Read the model definition and answer for the solid it produces. Units are mm, in the model's axes. A direction names the side the tool comes from. Give positions to 0.01 mm unless a question says otherwise; leave off trailing zeros. Write each loop counter-clockwise with the first axis right and the second up, starting at its lowest first coordinate (ties: lowest second). Pieces come first, ordered by that corner, then holes. Notation, with made-up numbers: M 17,71.25 L 52,71.25 A16 ccw 52,84.25 Z; hole C -6,12 d6. An arc over 180 degrees is marked long. Use a Markdown table: item, result. Add a question column.
Item 1: A cutting plane is placed at C-C on y = 28. Determine the outline of the cut face in (x, z) (3 decimals), then the cut area to 3 significant figures.
Item 2: For faces 1 (the flat face through (-40.64, 0, 19)), 2 (the flat face through (48, 12.7, 19)), 3 (the flat face through (62.23, 21, 19)), 4 (the flat face through (-55, 3.175, 19)), 5 (the cylindrical face through (-62.68, 8.18, 26.34)), determine the directions among +Z, -Z, +X, -X, +Y, -Y from which every point of the face is accessible in a straight line to the end or side of a thin tool.
Item 3: Consider probe 1 along X at (y, z) = (-6, 8.5) (3 decimals); probe 2 along Y at (x, z) = (0.5, 3.5) (3 decimals); probe 3 along X at (y, z) = (8.5, 27). Determine where each line is inside the solid, lowest interval first. Write a range as [from, to].
Item 4: The mould has two halves that part along X. Classify faces 6 (the flat face through (2, -17.78, 19)), 7 (the flat face through (1, -27.305, 19)), 8 (the flat face through (-50.165, -5, 19)): pulls with the +X half, pulls with the -X half, needs draft (parallel to the pull), parting line crosses it, or undercut.
Item 5: A cutting plane is placed at A-A on z = 23.5. Determine the outline of the cut face in (x, y) (1 decimal), then the cut area to 3 significant figures.
Item 6: Given P1, Ø4, axis at x = -64.14, z = 18.98, coming from the +Y side; P2, Ø7.5, axis at y = -1, z = 28, coming from the -X side (3 decimals); P3, Ø12.5, axis at y = -5, z = 25, coming from the +X side, each flat-ended and moving along its own axis, determine where each tip first touches the part or whether it passes through.
Item 7: A cutting plane is placed at D-D on x = -30.5. Determine the outline of the cut face in (y, z) (3 decimals), then the cut area to 3 significant figures.
Item 8: A cutting plane is placed at B-B on z = 31.75. Determine the outline of the cut face in (x, y) (1 decimal), then the cut area to 3 significant figures.
from build123d import *

# Parameters (mm, degrees)
BOSS_EXTRUDE1_DEPTH = 38.1
FILLET1_R           = 2.54
FILLET2_R           = 10.16
CUT_EXTRUDE2_DEPTH  = 91.653895256
SKETCH3_R           = 1.5875
CUT_EXTRUDE3_DEPTH  = 145.905274749
SKETCH4_R           = 1.5875
CUT_EXTRUDE4_DEPTH  = 91.653895347


with BuildPart() as part:
    # Sketch1 → Boss-Extrude1 (new body)
    with BuildSketch(Plane.XY):
        with BuildLine():
            Line((-35.8775, -27.305), (38.4175, -27.305))
            ThreePointArc((38.4175, -27.305), (48.520288136, -23.120288136), (52.705, -13.0175))
            Line((52.705, -13.0175), (52.705, -1.5875))
            ThreePointArc((52.705, -1.5875), (54.099903955, 1.780096045), (57.4675, 3.175))
            Line((57.4675, 3.175), (62.23, 3.175))
            Line((62.23, 3.175), (62.23, 47.625))
            Line((62.23, 47.625), (52.705, 47.625))
            Line((52.705, 47.625), (52.705, 12.7))
            Line((52.705, 12.7), (43.18, 12.7))
            Line((43.18, 12.7), (43.18, -13.0175))
            ThreePointArc((43.18, -13.0175), (41.785096045, -16.385096045), (38.4175, -17.78))
            Line((38.4175, -17.78), (-35.8775, -17.78))
            ThreePointArc((-35.8775, -17.78), (-39.245096045, -16.385096045), (-40.64, -13.0175))
            Line((-40.64, -13.0175), (-40.64, 12.7))
            Line((-40.64, 12.7), (-50.165, 12.7))
            Line((-50.165, 12.7), (-59.69, 12.7))
            Line((-59.69, 12.7), (-69.215, 12.7))
            Line((-69.215, 12.7), (-69.215, 3.175))
            Line((-69.215, 3.175), (-50.165, 3.175))
            Line((-50.165, 3.175), (-50.165, -13.0175))
            ThreePointArc((-50.165, -13.0175), (-45.980288136, -23.120288136), (-35.8775, -27.305))
        make_face()
    extrude(amount=BOSS_EXTRUDE1_DEPTH)

    # Fillet1
    fillet1_edges = [part.edges().sort_by_distance(p)[0] for p in [
        (62.23, 3.175, 19.05),
    ]]
    fillet(fillet1_edges, radius=FILLET1_R)

    # Fillet2
    # the kernel refuses this fillet: 10.16 mm, written as the material it takes off along each edge
    with BuildSketch(Plane(origin=(-69.215, 3.175, -25.350342083), x_dir=(1, 0, 0), z_dir=(0, 0, 1))) as fillet2_piece_1:
        with BuildLine():
            CenterArc((10.140136833, 10.16), FILLET2_R, 183.583321698, 86.416678302)
            Line((0, 9.525), (-0.202802737, 9.5123))
            ThreePointArc((-0.202802737, 9.5123), (-0.2032, 4.7625), (-0.2032, 0))
            Line((-0.2032, 0), (0, -0.2032))
            Line((0, -0.2032), (10.140136833, -0.2032))
            Line((10.140136833, -0.2032), (10.140136833, 0))
        make_face()
    extrude(amount=88.800684167, mode=Mode.SUBTRACT)
    with BuildSketch(Plane(origin=(62.23, 47.625, -25.350342083), x_dir=(0, -1, 0), z_dir=(0, 0, 1))) as fillet2_piece_2:
        with BuildLine():
            CenterArc((10.140136833, -10.16), FILLET2_R, 90, 86.416678302)
            Line((0, -9.525), (-0.202802737, -9.5123))
            ThreePointArc((-0.202802737, -9.5123), (-0.2032, -4.7625), (-0.2032, 0))
            Line((-0.2032, 0), (0, 0.2032))
            Line((0, 0.2032), (10.140136833, 0.2032))
            Line((10.140136833, 0.2032), (10.140136833, 0))
        make_face()
    extrude(amount=88.800684167, mode=Mode.SUBTRACT)

    # Sketch2 → Cut-Extrude2 (cut, through all)
    with BuildSketch(Plane.XZ.offset(-3.175)):
        Polygon((-69.215, -5.08), (-50.165, -5.08), (-69.215, 19.05), align=None)
    extrude(amount=-CUT_EXTRUDE2_DEPTH, mode=Mode.SUBTRACT)

    # Sketch3 → Cut-Extrude3 (cut, through all)
    with BuildSketch(Plane(origin=(62.23, 0, 0), x_dir=(0, 0, -1), z_dir=(1, 0, 0))):
        with Locations((-6.35, 42.554931583)):
            Circle(SKETCH3_R)
        with Locations((-19.05, 42.554931583)):
            Circle(SKETCH3_R)
        with Locations((-31.75, 42.554931583)):
            Circle(SKETCH3_R)
    extrude(amount=-CUT_EXTRUDE3_DEPTH, mode=Mode.SUBTRACT)

    # Sketch4 → Cut-Extrude4 (cut, through all)
    with BuildSketch(Plane.XZ.offset(-3.175)):
        with Locations((-64.144931583, 34.925)):
            Circle(SKETCH4_R)
        with Locations((-64.144931583, 26.951456669)):
            Circle(SKETCH4_R)
        with Locations((-64.144931583, 18.977913339)):
            Circle(SKETCH4_R)
    extrude(amount=-CUT_EXTRUDE4_DEPTH, mode=Mode.SUBTRACT)


solid = part.part
Filled in:
| question | item | result |
|---|---|---|
| 1 | outline | M 52.705,0 L 62.23,0 L 62.23,38.1 L 52.705,38.1 Z |
| 1 | area | 363 mm² |
| 2 | face 1 | +Z, -Z, +Y |
| 2 | face 2 | +Z, -Z, -X, +Y |
| 2 | face 3 | +Z, -Z, +X, +Y, -Y |
| 2 | face 4 | +Z, -Z, -X, -Y |
| 2 | face 5 | +Y, -Y |
| 3 | probe 1 | [-50.165, -40.64], [43.18, 52.705] |
| 3 | probe 2 | [-27.305, -17.78] |
| 3 | probe 3 | [-68.01, -65.73], [-62.56, -40.64], [43.18, 62.23] |
| 4 | face 6 | undercut |
| 4 | face 7 | needs draft |
| 4 | face 8 | pulls with the -X half |
| 5 | outline | M -69.2,12.7 A10.2 ccw -59.1,3.2 L -50.2,3.2 L -50.2,-13 A14.3 ccw -35.9,-27.3 L 38.4,-27.3 A14.3 ccw 52.7,-13 L 52.7,-1.6 A4.8 cw 57.5,3.2 L 59.7,3.2 A2.5 ccw 62.2,5.7 L 62.2,37.5 A10.2 ccw 52.7,47.6 L 52.7,12.7 L 43.2,12.7 L 43.2,-13 A4.8 cw 38.4,-17.8 L -35.9,-17.8 A4.8 cw -40.6,-13 L -40.6,12.7 Z |
| 5 | area | 2,050 mm² |
| 6 | P1 | y = 12.7 |
| 6 | P2 | x = -50.165 |
| 6 | P3 | x = 53.64 |
| 7 | outline | M -27.305,0 L -17.78,0 L -17.78,38.1 L -27.305,38.1 Z |
| 7 | area | 363 mm² |
| 8 | outline | M -69.2,12.7 A10.2 ccw -59.1,3.2 L -50.2,3.2 L -50.2,-13 A14.3 ccw -35.9,-27.3 L 38.4,-27.3 A14.3 ccw 52.7,-13 L 52.7,-1.6 A4.8 cw 57.5,3.2 L 59.7,3.2 A2.5 ccw 62.2,5.7 L 62.2,37.5 A10.2 ccw 61.6,41 L 52.7,41 L 52.7,12.7 L 43.2,12.7 L 43.2,-13 A4.8 cw 38.4,-17.8 L -35.9,-17.8 A4.8 cw -40.6,-13 L -40.6,12.7 Z; M 52.7,44.1 L 59.7,44.1 A10.2 ccw 52.7,47.6 Z |
| 8 | area | 2,020 mm² |
